Verification items for the finished model (mm, model axes). A direction names the side the tool comes from. Round coordinates to 2 decimals unless told otherwise and drop trailing zeros. Write each loop counter-clockwise with the first axis right and the second up, starting at its lowest first coordinate (ties: lowest second). Pieces come first, ordered by that corner, then holes. Notation, with made-up numbers: (-37.5, 26) - (-8.5, 26) arc R31 ccw to (-8.5, 53) - close; hole circle Ø7 at (-12, 47). An arc over 180 degrees is marked (long way). Answer as a JSON object with one key per item and string values. Group by question number.
1) Thickness scan on line 1 (X direction, y = 0, z = 0.15); line 2 (Z direction, x = 3.25, y = 11); line 3 (X direction, y = -0.5, z = 9). Record the ranges inside material, lowest first.
2) Set-up check for faces 4 (the flat face through (8, 0, 0.45)), 5 (the flat face through (9, 11, 24.9)), 6 (the flat face through (0, 0, 40.4)): record each of +Z, -Z, +X, -X, +Y, -Y from which the full face is reachable in a straight line by a thin tool's end or side.
3) Mould release check, pull along X, two halves, no side actions. Record for faces 1 (the flat face through (1, 1, -2.6)), 2 (the cylindrical face through (-0.91, 0.7, -9.4)), 3 (the cylindrical face through (9.24, -0.39, 0.22)): +X half, -X half, draft (parallel to the pull), parting line (faces both ways), or undercut.
4) Section check D-D (y = -3.75). Enter the section's corners in (x, z), then the cut area to 3 significant figures.
5) Section check A-A (x = 0). Enter the section's corners in (y, z).
6) Section check C-C (z = 25.5). Enter the section's corners in (x, y).
7) Go/stop test with flat-tipped pins: pin 1 Ø4 at (x, y) = (-3.5, -10) entering from -Z; pin 2 Ø1.5 at (y, z) = (2.5, 1) entering from -X; pin 3 Ø2.5 at (x, y) = (8, 0) entering from +Z. Record where each tip stops, or that it passes through.
```python
from build123d import *

# Parameters (mm, degrees)
SKETCH_R     = 13.85
PAD_DEPTH    = 37.8
SKETCH001_R  = 14.6
PAD001_DEPTH = 20
SKETCH002_R  = 5
PAD002_DEPTH = 2.6
SKETCH003_R  = 1.15
PAD003_DEPTH = 16.4
SKETCH004_R  = 5
PAD004_DEPTH = 2.6
SKETCH005_R  = 1.3
POCKET_DEPTH = 0.45


with BuildPart() as part:
    # Sketch → Pad (new body)
    with BuildSketch(Plane.XY):
        Circle(SKETCH_R)
    extrude(amount=PAD_DEPTH)

    # Sketch001 (on Face3 of Pad) → Pad001 (join)
    with BuildSketch(Plane.XY.offset(4.9)):
        Circle(SKETCH001_R)
    extrude(amount=PAD001_DEPTH)

    # Sketch002 (on Face7 of Pad001) → Pad002 (join)
    with BuildSketch(Plane.XY.offset(37.8)):
        Circle(SKETCH002_R)
    extrude(amount=PAD002_DEPTH)

    # Sketch003 (on Face2 of Pad002) → Pad003 (join)
    with BuildSketch(Plane(origin=(0, 0, 0), x_dir=(1, 0, 0), z_dir=(0, 0, -1))):
        Circle(SKETCH003_R)
    extrude(amount=PAD003_DEPTH)

    # Sketch004 (on Face2 of Pad003) → Pad004 (join)
    with BuildSketch(Plane(origin=(0, 0, 0), x_dir=(1, 0, 0), z_dir=(0, 0, -1))):
        Circle(SKETCH004_R)
    extrude(amount=PAD004_DEPTH)

    # Sketch005 (on Face2 of Pad004) → Pocket (cut)
    with BuildSketch(Plane(origin=(0, 0, 0), x_dir=(1, 0, 0), z_dir=(0, 0, -1))):
        with Locations((8, 0)):
            Circle(SKETCH005_R)
        with Locations((-8, 0)):
            Circle(SKETCH005_R)
    extrude(amount=-POCKET_DEPTH, mode=Mode.SUBTRACT)


solid = part.part
```
Returned:
{
 "1": {"line 1": "-13.85 to -9.3, -6.7 to 6.7, 9.3 to 13.85", "line 2": "0 to 37.8", "line 3": "-14.59 to 14.59"},
 "2": {"face 4": "-Z", "face 5": "+Z", "face 6": "+Z, +X, -X, +Y, -Y"},
 "3": {"face 1": "draft", "face 2": "parting line", "face 3": "undercut"},
 "4": {"outline": "(-14.11, 4.9) - (-13.33, 4.9) - (-13.33, 0) - (-3.31, 0) - (-3.31, -2.6) - (3.31, -2.6) - (3.31, 0) - (13.33, 0) - (13.33, 4.9) - (14.11, 4.9) - (14.11, 24.9) - (13.33, 24.9) - (13.33, 37.8) - (3.31, 37.8) - (3.31, 40.4) - (-3.31, 40.4) - (-3.31, 37.8) - (-13.33, 37.8) - (-13.33, 24.9) - (-14.11, 24.9) - close", "area": "1,070 mm2"},
 "5": {"outline": "(-14.6, 4.9) - (-13.85, 4.9) - (-13.85, 0) - (-5, 0) - (-5, -2.6) - (-1.15, -2.6) - (-1.15, -16.4) - (1.15, -16.4) - (1.15, -2.6) - (5, -2.6) - (5, 0) - (13.85, 0) - (13.85, 4.9) - (14.6, 4.9) - (14.6, 24.9) - (13.85, 24.9) - (13.85, 37.8) - (5, 37.8) - (5, 40.4) - (-5, 40.4) - (-5, 37.8) - (-13.85, 37.8) - (-13.85, 24.9) - (-14.6, 24.9) - close"},
 "6": {"outline": "circle Ø27.7 at (0, 0)"},
 "7": {"pin 1": "z = 0", "pin 2": "x = -13.74", "pin 3": "z = 37.8"}
}
